The listing builds one solid part. Answer for the finished solid, in the listing's coordinates (mm). A direction names the side the tool comes from. Coordinates: 2 decimals unless noted, no trailing zeros. Order: outer loops, then holes, each group sorted by start corner. A loop starts at its lowest first (then second) coordinate and runs counter-clockwise, first axis right, second up. Notation, with made-up numbers: (52, -26.5) -> (83, -26.5) arc R12 ccw to (83, -13.5) -> close; hole circle Ø5 at (58.5, 0.5). An arc over 180 degrees is marked (long way). Write item = value, one per line. Start each with the question number.
```python
from build123d import *

# Parameters (mm, degrees)
SKETCH1_R           = 31.685
SKETCH1_R_2         = 29.685
BOSS_EXTRUDE1_DEPTH = 50
SKETCH2_R           = 34
SKETCH2_R_2         = 29.685
BOSS_EXTRUDE2_DEPTH = 1
FILLET1_R           = 10


with BuildPart() as part:
    # Sketch1 → Boss-Extrude1 (new, symmetric)
    with BuildSketch(Plane.XY):
        Circle(SKETCH1_R)
        Circle(SKETCH1_R_2, mode=Mode.SUBTRACT)
    extrude(amount=BOSS_EXTRUDE1_DEPTH, both=True)

    # Sketch2 → Boss-Extrude2 (add, symmetric)
    with BuildSketch(Plane.XY.offset(19)):
        Circle(SKETCH2_R)
        Circle(SKETCH2_R_2, mode=Mode.SUBTRACT)
    extrude(amount=BOSS_EXTRUDE2_DEPTH, both=True)

    # Fillet1
    # the kernel refuses this fillet: 10 mm, written as the material it takes off along each edge
    with BuildSketch(Plane(origin=(0, 0, -50), x_dir=(1, 0, 0), z_dir=(0, -1, 0))) as fillet1_piece_1:
        with BuildLine():
            CenterArc((21.685, 6), FILLET1_R, 323.130102354, 36.869897646)
            Line((29.685, 0), (29.845, -0.12))
            ThreePointArc((29.845, -0.12), (30.685, -0.2), (31.685, -0.2))
            Line((31.685, -0.2), (31.885, 0))
            Line((31.885, 0), (31.885, 6))
            Line((31.885, 6), (31.685, 6))
        make_face()
    revolve(axis=Axis((0, 0, -50), (0, 0, 1)), mode=Mode.SUBTRACT)
    with BuildSketch(Plane(origin=(0, 0, 50), x_dir=(1, 0, 0), z_dir=(0, -1, 0))) as fillet1_piece_2:
        with BuildLine():
            CenterArc((39.685, -6), FILLET1_R, 143.130102354, 36.869897646)
            Line((31.685, 0), (31.525, 0.12))
            ThreePointArc((31.525, 0.12), (30.685, 0.2), (29.685, 0.2))
            Line((29.685, 0.2), (29.485, 0))
            Line((29.485, 0), (29.485, -6))
            Line((29.485, -6), (29.685, -6))
        make_face()
    revolve(axis=Axis((0, 0, 50), (0, 0, 1)), mode=Mode.SUBTRACT)


solid = part.part
```
Item 1: For a pull along Y with two mould halves and no side action, classify faces 3 (the cylindrical face through (-3.864, 29.432, -3.658)), 4 (the cylindrical face through (30.22, 9.52, -12.57)), 5 (the flat face through (23, -23, 18)) as pulls with the +Y half, pulls with the -Y half, needs draft (parallel to the pull), parting line crosses it, or undercut.
Item 2: Consider probe 1 along Y at (x, z) = (0, 9) (3 decimals); probe 2 along X at (y, z) = (-0.5, -11.5); probe 3 along Y at (x, z) = (17, 21.5). Determine where each line is inside the solid, lowest interval first.
Item 3: Which of the six approach directions +Z, -Z, +X, -X, +Y, -Y give full straight-line access (tool end or side, diameter ignored) to faces 1 (the flat face through (23, -23, 20)), 2 (the cylindrical face through (18.28, 28.67, 19.01))?
Item 4: Section C-C, the plane z = 11.5 is taken. Give the vertices of the cut face in (x, y) (3 decimals), then the cut area to 3 significant figures.
Item 5: Each of these flat-tipped pins is pushed along its axis until it touches: pin 1 (1.5 mm diameter, centred on x = 1, z = 16, fed in from +Y); pin 2 (4 mm diameter, centred on y = 5, z = -33, fed in from +X); pin 3 (8 mm diameter, centred on x = 21.5, z = 16, fed in from -Y). Where does it stop, or does it pass through?
Item 6: Section A-A, the plane x = 0 is taken. Give the vertices of the cut face in (y, z) (3 decimals).
A:
q1.face_3 = undercut
q1.face_4 = parting line crosses it
q1.face_5 = needs draft
q2.probe_1 = -31.685 to -29.685, 29.685 to 31.685
q2.probe_2 = -31.68 to -29.68, 29.68 to 31.68
q2.probe_3 = -26.74 to -24.34, 24.34 to 26.74
q3.face_1 = +Z
q3.face_2 = +Z, -Z
q4.outline = circle Ø63.37 at (0, 0); hole circle Ø59.37 at (0, 0)
q4.area = 386 mm^2
q5.pin_1 = 31.68
q5.pin_2 = 31.54
q5.pin_3 = -28.82
q6.outline = (-34, 18) -> (-31.685, 18) -> (-31.685, -44) arc R10 ccw to (-29.685, -50) -> (-29.685, 44) arc R10 ccw to (-31.685, 50) -> (-31.685, 20) -> (-34, 20) -> close; (29.685, -50) arc R10 ccw to (31.685, -44) -> (31.685, 18) -> (34, 18) -> (34, 20) -> (31.685, 20) -> (31.685, 50) arc R10 ccw to (29.685, 44) -> close
